Source: CAD feature listing. Evaluate the final solid. Frame: model axes, mm. A direction names the side the tool comes from. Give positions to 0.01 mm unless a question says otherwise; leave off trailing zeros. Write each loop counter-clockwise with the first axis right and the second up, starting at its lowest first coordinate (ties: lowest second). Pieces come first, ordered by that corner, then holes. Notation, with made-up numbers: M 30.5,34 L 75.5,34 A24 cw 75.5,56 Z; hole C -2,-29.75 d5. An arc over 180 degrees is marked long. Return JSON: item names as keys, results as strings.
```python
from build123d import *

# Parameters (mm, degrees)
SKETCH1_R                 = 1.651
BOSS_EXTRUDE2_DEPTH       = 5.3975
SKETCH2_R                 = 1.143
CUT_EXTRUDE1_DEPTH        = 6.3975
SKETCH3_R                 = 12.1285
CUT_EXTRUDE2_DEPTH        = 6.3975
SKETCH4_W                 = 28.562713242
SKETCH4_H                 = 11.677503754
BOSS_EXTRUDE3_DEPTH       = 5.3975
SKETCH5_W                 = 230.699333954
SKETCH5_H                 = 107.587024537
CUT_EXTRUDE3_DEPTH        = 6.3975
SKETCH6_R                 = 12.1285
CUT_EXTRUDE4_DEPTH        = 6.3975
SKETCH156_W               = 11.43
SKETCH156_H               = 10.16
CUT_EXTRUDE152_DEPTH      = 6.3975
SKETCH212_R               = 1.651
CUT_EXTRUDE208_DEPTH      = 97.79
SKETCH266_R               = 3.175
CUT_EXTRUDE262_DEPTH      = 103.378
CUT_EXTRUDE262_DEPTH_BACK = 48.768
CUT_EXTRUDE155_DEPTH      = 26.162
FILLET1_R                 = 2.54


with BuildPart() as part:
    # Sketch1 → Boss-Extrude2 (new body)
    with BuildSketch(Plane.XY):
        with BuildLine():
            Line((-65.2537815, 36.83), (-54.8397815, 36.83))
            Line((-54.8397815, 36.83), (-54.8397815, -36.83))
            Line((-54.8397815, -36.83), (-65.2537815, -36.83))
            ThreePointArc((-65.2537815, -36.83), (0, -74.93), (65.2537815, -36.83))
            Line((65.2537815, -36.83), (54.8397815, -36.83))
            Line((54.8397815, -36.83), (54.8397815, 36.83))
            Line((54.8397815, 36.83), (65.2537815, 36.83))
            ThreePointArc((65.2537815, 36.83), (0, 74.93), (-65.2537815, 36.83))
        make_face()
        with Locations((-45.466, 11.049)):
            Circle(SKETCH1_R, mode=Mode.SUBTRACT)
        with Locations((-20.067270032, 10.795)):
            Circle(SKETCH1_R, mode=Mode.SUBTRACT)
        with Locations((-20.067270032, -10.795)):
            Circle(SKETCH1_R, mode=Mode.SUBTRACT)
        with Locations((-45.466, -11.049)):
            Circle(SKETCH1_R, mode=Mode.SUBTRACT)
        with Locations((45.466, -11.049)):
            Circle(SKETCH1_R, mode=Mode.SUBTRACT)
        with Locations((20.067270032, -10.795)):
            Circle(SKETCH1_R, mode=Mode.SUBTRACT)
        with Locations((20.067270032, 10.795)):
            Circle(SKETCH1_R, mode=Mode.SUBTRACT)
        with Locations((45.466, 11.049)):
            Circle(SKETCH1_R, mode=Mode.SUBTRACT)
    extrude(amount=BOSS_EXTRUDE2_DEPTH)

    # Sketch2 → Cut-Extrude1 (cut, through all)
    with BuildSketch(Plane.XY.offset(5.3975)):
        with Locations((-6.731, 62.23)):
            Circle(SKETCH2_R)
        with Locations((6.731, 62.23)):
            Circle(SKETCH2_R)
    extrude(amount=-CUT_EXTRUDE1_DEPTH, mode=Mode.SUBTRACT)

    # Sketch3 → Cut-Extrude2 (cut, through all)
    with BuildSketch(Plane(origin=(0, 0, 0), x_dir=(-1, 0, 0), z_dir=(0, 0, -1))):
        with Locations((-42.926, -42.926)):
            Circle(SKETCH3_R)
        with Locations((13.97, -34.29)):
            Circle(SKETCH3_R)
        with Locations((13.97, 34.29)):
            Circle(SKETCH3_R)
        with Locations((-42.926, 42.926)):
            Circle(SKETCH3_R)
        with Locations((42.926, 42.926)):
            Circle(SKETCH3_R)
        with Locations((-13.97, 34.29)):
            Circle(SKETCH3_R)
        with Locations((-13.97, -34.29)):
            Circle(SKETCH3_R)
        with Locations((42.926, -42.926)):
            Circle(SKETCH3_R)
    extrude(amount=-CUT_EXTRUDE2_DEPTH, mode=Mode.SUBTRACT)

    # Sketch4 → Boss-Extrude3 (add)
    with BuildSketch(Plane(origin=(0, 0, 0), x_dir=(-1, 0, 0), z_dir=(0, 0, -1))):
        with Locations((-1.488809975, 62.152540216)):
            Rectangle(SKETCH4_W, SKETCH4_H)
    extrude(amount=-BOSS_EXTRUDE3_DEPTH)

    # Sketch5 → Cut-Extrude3 (cut, through all)
    with BuildSketch(Plane(origin=(0, 0, 0), x_dir=(-1, 0, 0), z_dir=(0, 0, -1))):
        with Locations((1.971047261, -36.648512269)):
            Rectangle(SKETCH5_W, SKETCH5_H)
    extrude(amount=-CUT_EXTRUDE3_DEPTH, mode=Mode.SUBTRACT)

    # Sketch6 → Cut-Extrude4 (cut, through all)
    with BuildSketch(Plane(origin=(0, 0, 0), x_dir=(-1, 0, 0), z_dir=(0, 0, -1))):
        with Locations((-15.777608989, 58.882838371)):
            Circle(SKETCH6_R)
        with Locations((15.777608989, 58.882838371)):
            Circle(SKETCH6_R)
    extrude(amount=-CUT_EXTRUDE4_DEPTH, mode=Mode.SUBTRACT)

    # Sketch156 → Cut-Extrude152 (cut, through all)
    with BuildSketch(Plane(origin=(0, 0, 0), x_dir=(-1, 0, 0), z_dir=(0, 0, -1))):
        with Locations((33.8847815, 22.225)):
            Rectangle(SKETCH156_W, SKETCH156_H)
        with Locations((-33.8847815, 22.225)):
            Rectangle(SKETCH156_W, SKETCH156_H)
    extrude(amount=-CUT_EXTRUDE152_DEPTH, mode=Mode.SUBTRACT)

    # Sketch212 → Cut-Extrude208 (cut)
    with BuildSketch(Plane(origin=(30.092005081, 4.08352975, -19.2405), x_dir=(-1, 0, 0), z_dir=(0, 0, -1))):
        with Locations((4.154396091, 41.38247025)):
            Circle(SKETCH212_R)
        with Locations((56.02961407, 41.38247025)):
            Circle(SKETCH212_R)
    extrude(amount=-CUT_EXTRUDE208_DEPTH, mode=Mode.SUBTRACT)

    # Sketch266 → Cut-Extrude262 (cut, two sides)
    with BuildSketch(Plane(origin=(30.092005081, 4.08352975, 16.891), x_dir=(-1, 0, 0), z_dir=(0, 0, -1))) as cut_extrude262_sk:
        with Locations((-16.897994919, 21.31647025)):
            Circle(SKETCH266_R)
        with Locations((77.082005081, 21.31647025)):
            Circle(SKETCH266_R)
        with Locations((30.092005081, 21.31647025)):
            Circle(SKETCH266_R)
    extrude(amount=CUT_EXTRUDE262_DEPTH, mode=Mode.SUBTRACT)
    extrude(cut_extrude262_sk.sketch, amount=-CUT_EXTRUDE262_DEPTH_BACK, mode=Mode.SUBTRACT)

    # Sketch159 → Cut-Extrude155 (cut)
    with BuildSketch(Plane(origin=(0, 0, 0), x_dir=(-1, 0, 0), z_dir=(0, 0, -1))):
        with BuildLine():
            Line((12.7, 20.24), (8.888991966, 20.24))
            ThreePointArc((8.888991966, 20.24), (5.715, 23.495), (2.541008034, 20.24))
            Line((2.541008034, 20.24), (-2.541008034, 20.24))
            ThreePointArc((-2.541008034, 20.24), (-5.715, 23.495), (-8.888991966, 20.24))
            Line((-8.888991966, 20.24), (-12.7, 20.24))
            ThreePointArc((-12.7, 20.24), (-16.235533906, 11.704466094), (-7.7, 15.24))
            Line((-7.7, 15.24), (7.7, 15.24))
            ThreePointArc((7.7, 15.24), (16.235533906, 11.704466094), (12.7, 20.24))
        make_face()
    extrude(amount=-CUT_EXTRUDE155_DEPTH, mode=Mode.SUBTRACT)

    # Fillet1
    fillet1_edges = [part.edges().sort_by_distance(p)[0] for p in [
        (-39.5997815, 17.145, 2.69875),
        (-28.1697815, 17.145, 2.69875),
        (28.1697815, 17.145, 2.69875),
        (39.5997815, 17.145, 2.69875),
        (-17.322875188, 17.145, 2.69875),
        (17.322875188, 17.145, 2.69875),
        (8.888991966, 20.24, 2.69875),
        (2.541008034, 20.24, 2.69875),
        (-2.541008034, 20.24, 2.69875),
        (-8.888991966, 20.24, 2.69875),
    ]]
    fillet(fillet1_edges, radius=FILLET1_R)


solid = part.part
```
1) Contact query for flat-ended pins moving along their axis: pin 1 Ø2.5 at (y, z) = (23.5, 2) entering from +X; pin 2 Ø3 at (y, z) = (50, 3) entering from -X; pin 3 Ø12 at (x, y) = (26.5, 44.5) entering from -Z; pin 4 Ø2 at (x, z) = (-11.5, 2.5) entering from -Y. Output: stop coordinate, or through.
Numbers:
{"pin 1": "stops at x = 54.84", "pin 2": "stops at x = -57.12", "pin 3": "stops at z = 0", "pin 4": "stops at y = 20.24"}
2) Draft query along Y for faces 5 (the face through (-1, 46, 5.398)), 6 (the face through (-48.697, 28.077, 2.737)), 7 (the face through (27.445, 17.909, 2.737)). Return one class per face: released by +Y, released by -Y, zero draft, split by the parting line, or undercut.
Numbers:
{"face 5": "zero draft", "face 6": "undercut", "face 7": "released by -Y"}
3) Cut plane A-A, the plane x = -46.99. Return the cut outline in (y, z) (1 decimal).
Numbers:
{"outline": "M 17.1,0 L 22.2,0 L 22.2,5.4 L 17.1,5.4 Z; M 28.6,0 L 31.5,0 L 31.5,5.4 L 28.6,5.4 Z; M 54.4,0 L 58.4,0 L 58.4,5.4 L 54.4,5.4 Z"}
4) Line query: line 1 (Y direction, x = 44.5, z = 0.45) (3 decimals); line 2 (Y direction, x = -17.5, z = 2.85); line 3 (X direction, y = 51, z = 1.2). Output: solid intervals per line, ascending. Write a range as [from, to].
Numbers:
{"line 1": "y = [17.145, 23.43], [27.37, 30.9], [54.952, 60.285]", "line 2": "y = [17.5, 22.69], [45.89, 46.88], [70.89, 72.86]", "line 3": "x = [-54.9, -51.98], [-33.88, -25], [-6.56, 6.56], [25, 33.88], [51.98, 54.9]"}
5) Set-up query: faces 1 (the face through (-54.84, 27, 3)), 2 (the face through (-1.895, 20.621, 2.737)), 3 (the face through (-25.54, 37.93, 2.66)), 4 (the face through (60, 36.83, 3)). Return all of +Z, -Z, +X, -X, +Y, -Y with unobstructed straight access to the full face (end or side cutting, diameter ignored); none if empty.
Numbers:
{"face 1": "+Z, -Z, -X, -Y", "face 2": "+Z, -Z, -Y", "face 3": "+Z, -Z", "face 4": "+Z, -Z, +X, -Y"}
6) Cut plane B-B, the plane y = 48.5. Return the cut outline in (x, z), then the cut area to 3 significant figures.
Numbers:
{"outline": "M -57.12,0 L -53.7,0 L -53.7,5.4 L -57.12,5.4 Z; M -32.15,0 L -22.05,0 L -22.05,5.4 L -32.15,5.4 Z; M -9.51,0 L 9.51,0 L 9.51,5.4 L -9.51,5.4 Z; M 22.05,0 L 32.15,0 L 32.15,5.4 L 22.05,5.4 Z; M 53.7,0 L 57.12,0 L 57.12,5.4 L 53.7,5.4 Z", "area": "249 mm²"}
7) Cut plane D-D, the plane y = 66.5. Return the cut outline in (x, z), then the cut area to 3 significant figures.
Numbers:
{"outline": "M -34.53,0 L -25.22,0 L -25.22,5.4 L -34.53,5.4 Z; M -6.34,0 L 6.34,0 L 6.34,5.4 L -6.34,5.4 Z; M 25.22,0 L 34.53,0 L 34.53,5.4 L 25.22,5.4 Z", "area": "169 mm²"}
8) Cut plane C-C, the plane y = 25.4. Give the number of separate pieces and of enclosed holes in the cut face, then the cut area to 3 significant figures.
Numbers:
{"separate pieces": "8", "enclosed holes": "0", "area": "188 mm²"}
